Read the model definition and answer for the solid it produces. Units are mm, in the model's axes. A direction names the side the tool comes from. Round coordinates to 2 decimals unless told otherwise and drop trailing zeros. Order: outer loops, then holes, each group sorted by start corner. A loop starts at its lowest first (then second) coordinate and runs counter-clockwise, first axis right, second up. Notation, with made-up numbers: (39.25, 46) - (77.25, 46) arc R22 cw to (77.25, 65) - close; hole circle Ø10 at (56.5, -24). An arc over 180 degrees is marked (long way). One line per question, with ' | ' between items. Start each with the question number.
1) Flat-ended cylindrical pins translate along their axes: pin 1 (8 mm diameter, centred on y = -53.5, z = -12, fed in from -X); pin 2 (3.5 mm diameter, centred on x = 15.56, z = 15.56, fed in from +Y); pin 3 (4.5 mm diameter, centred on x = -15.5, z = -15.5, fed in from +Y). Find the tip coordinate at first contact, or state that the pin passes through.
2) The part is cut by section B-B, the plane x = 0. Give the vertices of the cut face in (y, z).
3) The mould has two halves that part along X. Classify faces 1 (the flat face through (0, 27, 0)), 2 (the conical face through (24.961, -0.486, 7.861)), 3 (the flat face through (16, -10, -16)): pulls with the +X half, pulls with the -X half, needs draft (parallel to the pull), parting line crosses it, or undercut.
4) The part is cut by section A-A, the plane z = 0. Give the vertices of the cut face in (x, y), plus the area to 3 significant figures.
5) For faces 4 (the cylindrical face through (-17.143, -4.93, -16.773)), 5 (the flat face through (0, -86, 0)), determine the directions among +Z, -Z, +X, -X, +Y, -Y from which every point of the face is accessible in a straight line to the end or side of a thin tool.
6) Straight lines are drawn through the part: line 1 (Y direction, x = 21, z = 6); line 2 (Z direction, x = 19, y = -77); line 3 (Z direction, x = 6, y = -3). For each, find the intervals that lie inside material, in ascending order. Write a range as from..to.
7) The part is cut by section C-C, the plane y = 8. Give the vertices of the cut face in (x, z).
from build123d import *

# Parameters (mm, degrees)
F0_R     = 29.5
F0_R_2   = 2
F0_R_3   = 4
F1_DEPTH = 86
F2_DEPTH = 27
F3_DEPTH = 10
F4_SIZE2 = 3.5
F4_SIZE  = 10
F5_SIZE2 = 10
F5_SIZE  = 3.5


with BuildPart() as f1:
    # F0 (on Front) → F1 (new body)
    with BuildSketch(Plane.XZ):
        Circle(F0_R)
        with Locations((-15.5563491861, -15.5563491861)):
            Circle(F0_R_2, mode=Mode.SUBTRACT)
        with Locations((15.5563491861, -15.5563491861)):
            Circle(F0_R_2, mode=Mode.SUBTRACT)
        with Locations((-15.5563491861, 15.5563491861)):
            Circle(F0_R_2, mode=Mode.SUBTRACT)
        Circle(F0_R_3, mode=Mode.SUBTRACT)
        with Locations((15.5563491861, 15.5563491861)):
            Circle(F0_R_2, mode=Mode.SUBTRACT)
        Circle(F0_R_3)
        with Locations((15.5563491861, 15.5563491861)):
            Circle(F0_R_2)
        with Locations((-15.5563491861, 15.5563491861)):
            Circle(F0_R_2)
        with Locations((-15.5563491861, -15.5563491861)):
            Circle(F0_R_2)
        with Locations((15.5563491861, -15.5563491861)):
            Circle(F0_R_2)
    extrude(amount=F1_DEPTH)

    # F0 (on Front) → F2 (join)
    with BuildSketch(Plane.XZ):
        Circle(F0_R_3)
    extrude(amount=-F2_DEPTH)

    # F0 (on Front) → F3 (cut)
    with BuildSketch(Plane.XZ):
        with Locations((15.5563491861, 15.5563491861)):
            Circle(F0_R_2)
        with Locations((-15.5563491861, 15.5563491861)):
            Circle(F0_R_2)
        with Locations((15.5563491861, -15.5563491861)):
            Circle(F0_R_2)
        with Locations((-15.5563491861, -15.5563491861)):
            Circle(F0_R_2)
    extrude(amount=F3_DEPTH, mode=Mode.SUBTRACT)

    # F4
    f4_edges = [f1.edges().sort_by_distance(p)[0] for p in [
        (-29.5, 0, 0),
    ]]
    f4_side = f1.faces().sort_by_distance((-29.5, -43, 0))[0]
    chamfer(f4_edges, length=F4_SIZE, length2=F4_SIZE2, reference=f4_side)

    # F5
    f5_edges = [f1.edges().sort_by_distance(p)[0] for p in [
        (-29.5, -86, 0),
    ]]
    f5_side = f1.faces().sort_by_distance((0, -86, 0))[0]
    chamfer(f5_edges, length=F5_SIZE, length2=F5_SIZE2, reference=f5_side)


solid = f1.part
Values:
1) pin 1: stops at x = -28.39 | pin 2: stops at y = -10 | pin 3: stops at y = 0
2) outline: (-86, -26) - (-76, -29.5) - (-10, -29.5) - (0, -26) - (0, -4) - (27, -4) - (27, 4) - (0, 4) - (0, 26) - (-10, 29.5) - (-76, 29.5) - (-86, 26) - close
3) face 1: needs draft | face 2: parting line crosses it | face 3: undercut
4) outline: (-29.5, -76) - (-26, -86) - (26, -86) - (29.5, -76) - (29.5, -10) - (26, 0) - (4, 0) - (4, 27) - (-4, 27) - (-4, 0) - (-26, 0) - (-29.5, -10) - close | area: 5,220 mm^2
5) face 4: +Y | face 5: +Z, -Z, +X, -X, -Y
6) line 1: y = -86..0 | line 2: z = -22.11..22.11 | line 3: z = -26.38..26.38
7) outline: circle Ø8 at (0, 0)
